Geometry check sheet. Reference: the model listing, model coordinates, mm. Face numbers are marked on the shaded views. Coordinates: 2 decimals unless noted, no trailing zeros. Write each loop counter-clockwise with the first axis right and the second up, starting at its lowest first coordinate (ties: lowest second). Pieces come first, ordered by that corner, then holes. Notation, with made-up numbers: (47, 60) -> (51, 60) arc R20 ccw to (51, 70) -> close; hole circle Ø11 at (24, 2). An arc over 180 degrees is marked (long way). One line per question, with ' | ' between items.
```python
from build123d import *

# Parameters (mm, degrees)
BASE_PCB_W              = 48
BASE_PCB_H              = 33
BASE_PCB_R              = 1.5
BOSS_EXTRU_1_DEPTH      = 1.6
ESQUISSE4_W             = 37.5
ESQUISSE4_H             = 32
BOSS_EXTRU_2_DEPTH      = 1.2
ESQUISSE5_W             = 27.6
ESQUISSE5_H             = 27.6
ENL_V_MAT_EXTRU_2_DEPTH = 0.5


with BuildPart() as part:
    # BASE PCB → Boss.-Extru.1 (new body)
    with BuildSketch(Plane.XY):
        Rectangle(BASE_PCB_W, BASE_PCB_H)
        with Locations((-21.5, 14)):
            Circle(BASE_PCB_R, mode=Mode.SUBTRACT)
        with Locations((-21.5, -14)):
            Circle(BASE_PCB_R, mode=Mode.SUBTRACT)
        with Locations(Location((21.5, -14, 0), (0, 0, 180))):
            Circle(BASE_PCB_R, mode=Mode.SUBTRACT)
        with Locations(Location((21.5, 14, 0), (0, 0, 180))):
            Circle(BASE_PCB_R, mode=Mode.SUBTRACT)
    extrude(amount=BOSS_EXTRU_1_DEPTH)

    # Esquisse4 → Boss.-Extru.2 (add)
    with BuildSketch(Plane.XY):
        Rectangle(ESQUISSE4_W, ESQUISSE4_H)
    extrude(amount=-BOSS_EXTRU_2_DEPTH)

    # Esquisse5 → Enlèv. mat.-Extru.2 (cut)
    with BuildSketch(Plane(origin=(0, 0, -1.2), x_dir=(-1, 0, 0), z_dir=(0, 0, -1))):
        with Locations((-2.95, 0)):
            Rectangle(ESQUISSE5_W, ESQUISSE5_H)
    extrude(amount=-ENL_V_MAT_EXTRU_2_DEPTH, mode=Mode.SUBTRACT)


solid = part.part
```
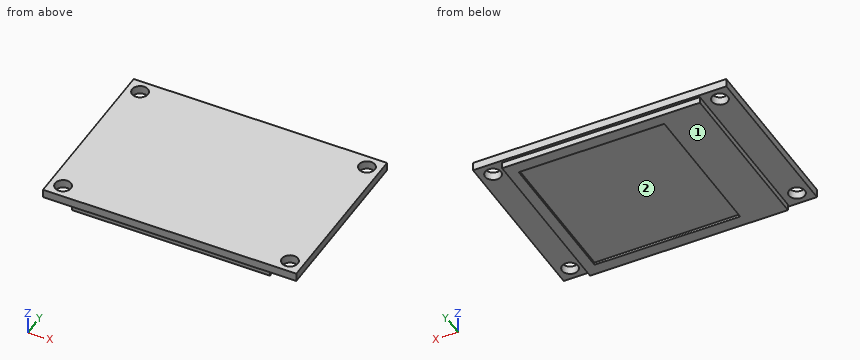
(1) Draft check along X on the marked faces 1 and 2. Enter one of: pulls with the +X half, pulls with the -X half, needs draft (parallel to the pull), parting line crosses it, or undercut.
Answers below:
face 1: needs draft | face 2: undercut
(2) Cross-section at A-A (x = 21.5). Record the cut outline in (y, z), plus the area to 3 significant figures.
Answers below:
outline: (-16.5, 0) -> (-15.5, 0) -> (-15.5, 1.6) -> (-16.5, 1.6) -> close; (-12.5, 0) -> (12.5, 0) -> (12.5, 1.6) -> (-12.5, 1.6) -> close; (15.5, 0) -> (16.5, 0) -> (16.5, 1.6) -> (15.5, 1.6) -> close | area: 43.2 mm²
(3) Cross-section at D-D (y = 12). Record the cut outline in (x, z).
Answers below:
outline: (-24, 0) -> (-18.75, 0) -> (-18.75, -1.2) -> (-10.85, -1.2) -> (-10.85, -0.7) -> (16.75, -0.7) -> (16.75, -1.2) -> (18.75, -1.2) -> (18.75, 0) -> (24, 0) -> (24, 1.6) -> (-24, 1.6) -> close
(4) Cross-section at C-C (x = -6.5). Record the cut outline in (y, z), plus the area to 3 significant figures.
Answers below:
outline: (-16.5, 0) -> (-16, 0) -> (-16, -1.2) -> (-13.8, -1.2) -> (-13.8, -0.7) -> (13.8, -0.7) -> (13.8, -1.2) -> (16, -1.2) -> (16, 0) -> (16.5, 0) -> (16.5, 1.6) -> (-16.5, 1.6) -> close | area: 77.4 mm²
(5) Cross-section at B-B (z = 0.8). Record the cut outline in (x, y), plus the area to 3 significant figures.
Answers below:
outline: (-24, -16.5) -> (24, -16.5) -> (24, 16.5) -> (-24, 16.5) -> close; hole circle Ø3 at (-21.5, -14); hole circle Ø3 at (-21.5, 14); hole circle Ø3 at (21.5, -14); hole circle Ø3 at (21.5, 14) | area: 1,560 mm²
(6) Material ranges on line 1 (Y direction, x = 21.5, z = 0.45); line 2 (Y direction, x = -21, z = 0.15); line 3 (X direction, y = -1, z = -1.1), recorded low to high.
Answers below:
line 1: y = -16.5 to -15.5, -12.5 to 12.5, 15.5 to 16.5 | line 2: y = -16.5 to -15.41, -12.59 to 12.59, 15.41 to 16.5 | line 3: x = -18.75 to -10.85, 16.75 to 18.75
(7) Depth check by flat-ended pin: P1, Ø1.3, axis at x = -2.5, z = -1, coming from the -Y side; P2, Ø4, axis at x = -21.5, y = -14, coming from the -Z side; P3, Ø3, axis at x = -19, y = 1.5, coming from the -Z side; P4, Ø0.6, axis at y = 0.5, z = -0.5, coming from the -X side. Enter the tip coordinate at first touch or a pass-through.
Answers below:
P1: stops at y = -16 | P2: stops at z = 0 | P3: stops at z = -1.2 | P4: stops at x = -18.75
